Verification items for this drawing (mm, ordinates from the low corner). A direction names the side the tool comes from. Round coordinates to 2 decimals unless told otherwise and drop trailing zeros. Loops run counter-clockwise (first coordinate to the right, second up) from the corner with the lowest first, then second, coordinate; pieces in that order, holes last. Notation, with made-up numbers: (-39, 38.25) - (9, 38.25) arc R19 cw to (9, 46.25) - close; hole circle Ø10 at (61, -6.75). An arc over 180 degrees is marked (long way). Answer in a Markdown table with one row per item. Add a question column.
(1) Cross-section at B-B on y = 41.5. Enter the section's corners in (x, z).
(2) Cross-section at A-A on z = 59.5. Enter the section's corners in (x, y).
(3) Thickness scan on line 1 along Z through (x, y) = (81, 29.5); line 2 along X through (y, z) = (25, 52.5); line 3 along Z through (x, y) = (27, 36). Record the ranges inside material, lowest first.
(4) Cross-section at D-D on y = 14. Enter the section's corners in (x, z).
(5) Gauge pin test, flat ends, axial feed: pin 1 (15.5 mm diameter, centred on x = 9, y = 27.5, fed in from -Z); pin 2 (9.5 mm diameter, centred on x = 5, z = 58, fed in from -Y); pin 3 (4 mm diameter, centred on y = 7, z = 29.5, fed in from -X). Record the tip position at first contact, or that the pin passes through.
(6) Access from +Z, -Z, +X, -X, +Y, -Y to the whole of each face (thin tool, end or side, straight path). Record for the marked faces 1, 2, 3 and 4.
(7) Cross-section at C-C on x = 89.5. Enter the section's corners in (y, z), then the cut area to 3 significant figures.
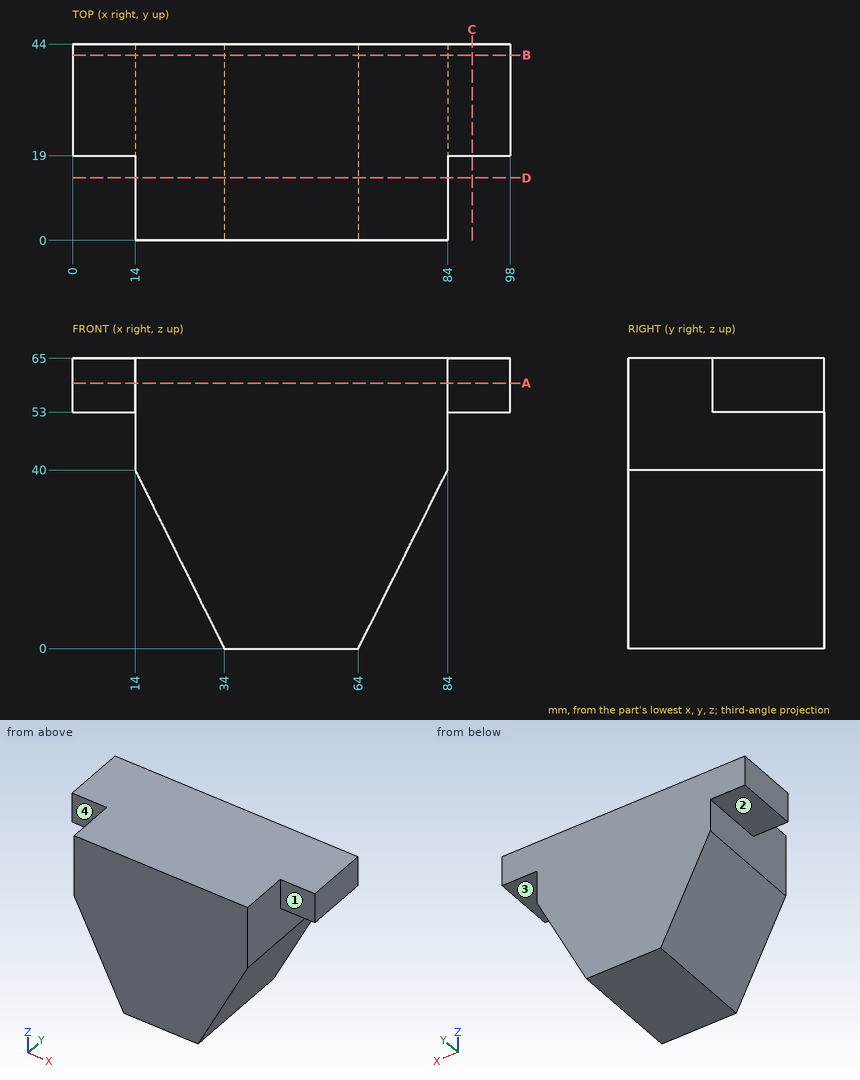
Answers:
| question | item | result |
|---|---|---|
| 1 | outline | (0, 53) - (14, 53) - (14, 40) - (34, 0) - (64, 0) - (84, 40) - (84, 53) - (98, 53) - (98, 65) - (0, 65) - close |
| 2 | outline | (0, 19) - (14, 19) - (14, 0) - (84, 0) - (84, 19) - (98, 19) - (98, 44) - (0, 44) - close |
| 3 | line 1 | z = 34 to 65 |
| 3 | line 2 | x = 14 to 84 |
| 3 | line 3 | z = 14 to 65 |
| 4 | outline | (14, 40) - (34, 0) - (64, 0) - (84, 40) - (84, 65) - (14, 65) - close |
| 5 | pin 1 | stops at z = 34.5 |
| 5 | pin 2 | stops at y = 19 |
| 5 | pin 3 | stops at x = 18.25 |
| 6 | face 1 | +Z, -Z, +X, -Y |
| 6 | face 2 | -Z, -X, +Y, -Y |
| 6 | face 3 | -Z, +X, +Y, -Y |
| 6 | face 4 | +Z, -Z, -X, -Y |
| 7 | outline | (19, 53) - (44, 53) - (44, 65) - (19, 65) - close |
| 7 | area | 300 mm^2 |
